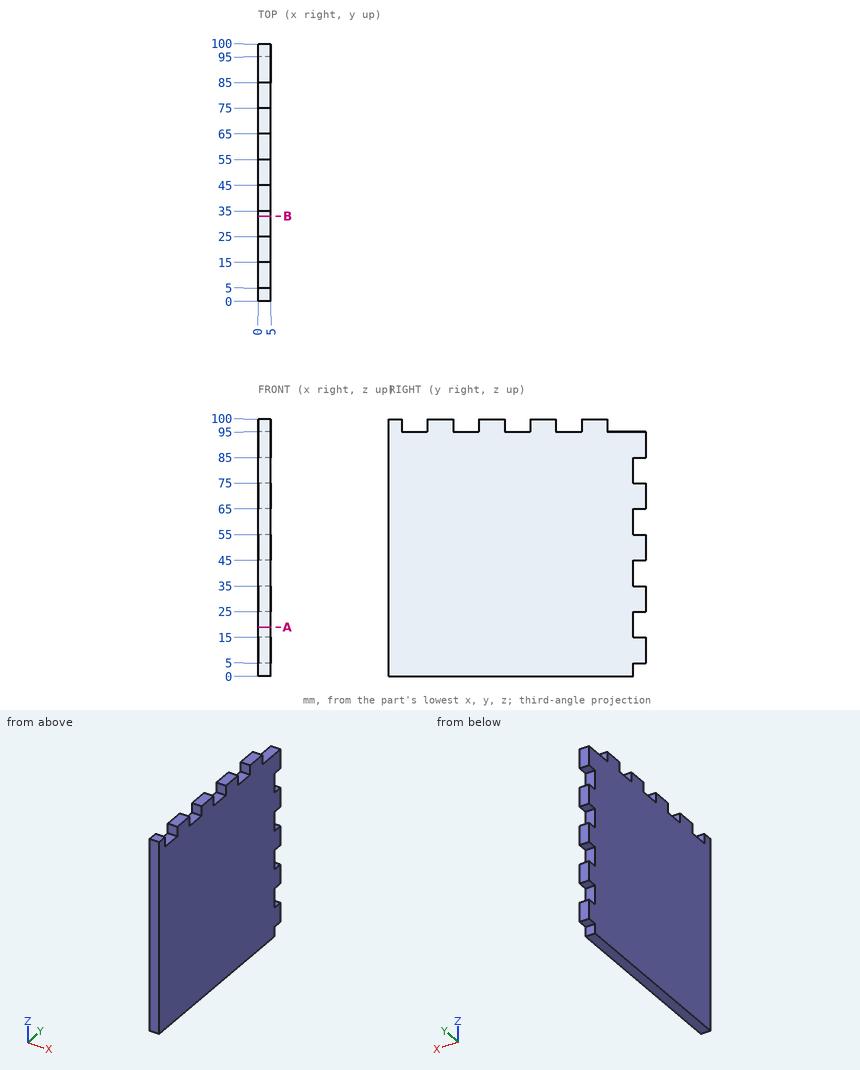
Print and shaded views of the part. All mm, measured from the part's lowest x, y and z. Coordinates: 2 decimals unless noted, no trailing zeros. Order: outer loops, then holes, each group sorted by start corner. A loop starts at its lowest first (then second) coordinate and runs counter-clockwise, first axis right, second up.
Item 1: Drop flat-ended pins along their axis: pin 1 Ø2.5 at (x, y) = (3.5, 29.5) entering from +Z; pin 2 Ø2.5 at (x, y) = (3, 96.5) entering from -Z; pin 3 Ø1.5 at (x, z) = (2.5, 81.5) entering from +Y. Give the stop position or say it passes through.
Filled in:
pin 1: stops at z = 95
pin 2: stops at z = 5
pin 3: stops at y = 95
Item 2: Drill centre line: L1, parallel to Z at x = 3.5, y = 94. Where is it in solid material? Low to high.
Filled in:
L1: z = 0 to 95
Item 3: Saw through at A-A on z = 19. List the corners of the cut face in (x, y).
Filled in:
outline: (0, 0) - (5, 0) - (5, 95) - (0, 95) - close
